The listing builds one solid part. Answer for the finished solid, in the listing's coordinates (mm). A direction names the side the tool comes from. Coordinates: 2 decimals unless noted, no trailing zeros. Write each loop counter-clockwise with the first axis right and the second up, starting at its lowest first coordinate (ties: lowest second). Pieces come first, ordered by that corner, then holes.
(1) For a pull along Y with two mould halves and no side action, classify faces 4 (the flat face through (22, 2, 5.1)), 5 (the flat face through (0, -15, 3)), 6 (the cylindrical face through (-35, 0, 3)) as +Y half, -Y half, draft (parallel to the pull), parting line (faces both ways), or undercut.
(2) Straight lines are drawn through the part: line 1 (Y direction, x = -20, z = 0.7); line 2 (X direction, y = -7, z = 4.2); line 3 (Y direction, x = 20, z = 2.15) (3 decimals). For each, find the intervals that lie inside material, in ascending order.
(3) Given P1, Ø10, axis at x = -20.5, y = 2.5, coming from the +Z side, flat-ended and moving along its own axis, determine where the tip first touches the part or whether it passes through.
(4) The part is cut by section B-B on y = -13. Determine the outline of the cut face in (x, z), plus the area to 3 significant figures.
(5) Which of the six approach directions +Z, -Z, +X, -X, +Y, -Y give full straight-line access (tool end or side, diameter ignored) to faces 1 (the flat face through (-7, 0, 0)), 2 (the cylindrical face through (-10.414, 3.019, 3.528)), 3 (the cylindrical face through (27.967, 0.351, 2.768))?
(6) The part is cut by section A-A on z = 2.2. Determine the outline of the cut face in (x, y) (3 decimals), plus the area to 3 significant figures.
from build123d import *

# Parameters (mm, degrees)
BOSS_EXTRUDE1_DEPTH = 6
SKETCH8_R           = 10.05
CUT_EXTRUDE4_DEPTH  = 4.5
SKETCH9_R           = 7.975
CUT_EXTRUDE5_DEPTH  = 5.1
SKETCH10_R          = 2.55
CUT_EXTRUDE6_DEPTH  = 1.9
SKETCH11_R          = 1.55
CUT_EXTRUDE7_DEPTH  = 2.5
CHAMFER1_SIZE       = 0.5


with BuildPart() as part:
    # Sketch4 → Boss-Extrude1 (new body)
    with BuildSketch(Plane.XY):
        with BuildLine():
            Line((-20, 15), (20, 15))
            ThreePointArc((20, 15), (35, 0), (20, -15))
            Line((20, -15), (-20, -15))
            ThreePointArc((-20, -15), (-35, 0), (-20, 15))
        make_face()
    extrude(amount=BOSS_EXTRUDE1_DEPTH)

    # Sketch8 → Cut-Extrude4 (cut)
    with BuildSketch(Plane.XY.offset(6)):
        with Locations((-20, 0)):
            Circle(SKETCH8_R)
    extrude(amount=-CUT_EXTRUDE4_DEPTH, mode=Mode.SUBTRACT)

    # Sketch9 → Cut-Extrude5 (cut)
    with BuildSketch(Plane(origin=(0, 0, 0), x_dir=(-1, 0, 0), z_dir=(0, 0, -1))):
        with Locations((-20, 0)):
            Circle(SKETCH9_R)
    extrude(amount=-CUT_EXTRUDE5_DEPTH, mode=Mode.SUBTRACT)

    # Sketch10 → Cut-Extrude6 (cut, through all)
    with BuildSketch(Plane(origin=(0, 0, 5.1), x_dir=(-1, 0, 0), z_dir=(0, 0, -1))):
        with Locations((-20, 0)):
            Circle(SKETCH10_R)
    extrude(amount=-CUT_EXTRUDE6_DEPTH, mode=Mode.SUBTRACT)

    # Sketch11 → Cut-Extrude7 (cut, through all)
    with BuildSketch(Plane.XY.offset(1.5)):
        with Locations((-20, 0)):
            Circle(SKETCH11_R)
        with Locations((-13, 0)):
            Circle(SKETCH11_R)
        with Locations((-27, 0)):
            Circle(SKETCH11_R)
        with Locations((-20, 7)):
            Circle(SKETCH11_R)
        with Locations((-20, -7)):
            Circle(SKETCH11_R)
    extrude(amount=-CUT_EXTRUDE7_DEPTH, mode=Mode.SUBTRACT)

    # Chamfer1
    chamfer1_edges = [part.edges().sort_by_distance(p)[0] for p in [
        (-30.05, 0, 6),
        (27.975, 0, 0),
    ]]
    chamfer(chamfer1_edges, length=CHAMFER1_SIZE)


solid = part.part
Model answer:
1. face 4: undercut
1. face 5: -Y half
1. face 6: parting line
2. line 1: y = -15 to -8.55, -5.45 to -1.55, 1.55 to 5.45, 8.55 to 15
2. line 2: x = -33.27 to -27.21, -12.79 to 16.18, 23.82 to 33.27
2. line 3: y = -15 to -7.975, 7.975 to 15
3. P1: stops at z = 1.5
4. outline: (-27.48, 0) - (27.48, 0) - (27.48, 6) - (-27.48, 6) - close
4. area: 330 mm2
5. face 1: -Z, +X, -X, +Y, -Y
5. face 2: +Z
5. face 3: -Z
6. outline: (-20, -15) - (20, -15) arc R15 ccw to (20, 15) - (-20, 15) arc R15 ccw to start; hole circle Ø20.1 at (-20, 0); hole circle Ø15.95 at (20, 0)
6. area: 1,390 mm2
